The listing builds one solid part. Answer for the finished solid, in the listing's coordinates (mm). A direction names the side the tool comes from. Give positions to 0.01 mm unless a question says otherwise; leave off trailing zeros. Write each loop counter-clockwise with the first axis right and the second up, starting at its lowest first coordinate (ties: lowest second). Pieces come first, ordered by that corner, then holes.
```python
from build123d import *

# Parameters (mm, degrees)
F1_DEPTH = 6
F2_R     = 6.25
F3_DEPTH = 3.5
F4_W     = 15.8
F4_H     = 32
F5_DEPTH = 4.5
F7_DEPTH = 32
F9_DEPTH = 15.8
F10_R    = 0.2


with BuildPart() as f1:
    # F0 (on Top) → F1 (new body)
    with BuildSketch(Plane.XY):
        with BuildLine():
            ThreePointArc((-29.927051, 63.999335), (-26.535898, 58), (-33.427051, 57.937157))
            Line((-33.427051, 57.937157), (-37.47822, 60.2761))
            ThreePointArc((-37.47822, 60.2761), (-38.509832, 60.257063), (-38.975497, 59.336334))
            ThreePointArc((-38.975497, 59.336334), (-38.676985, 57.610456), (-38.049845, 55.975078))
            Line((-38.049845, 55.975078), (-8.049845, -4.024922))
            ThreePointArc((-8.049845, -4.024922), (-6.775035, -5.924433), (-5.0625, -7.441176))
            ThreePointArc((-5.0625, -7.441176), (-4.032293, -7.498262), (-3.5, -6.614378))
            Line((-3.5, -6.614378), (-3.5, -1.936492))
            ThreePointArc((-3.5, -1.936492), (0, 4), (3.5, -1.936492))
            Line((3.5, -1.936492), (3.5, -6.614378))
            ThreePointArc((3.5, -6.614378), (4.032293, -7.498262), (5.0625, -7.441176))
            ThreePointArc((5.0625, -7.441176), (6.775035, -5.924433), (8.049845, -4.024922))
            Line((8.049845, -4.024922), (38.049845, 55.975078))
            ThreePointArc((38.049845, 55.975078), (38.676985, 57.610456), (38.975497, 59.336334))
            ThreePointArc((38.975497, 59.336334), (38.509832, 60.257063), (37.47822, 60.2761))
            Line((37.47822, 60.2761), (33.427051, 57.937157))
            ThreePointArc((33.427051, 57.937157), (26.535898, 58), (29.927051, 63.999335))
            Line((29.927051, 63.999335), (33.97822, 66.338278))
            ThreePointArc((33.97822, 66.338278), (34.477539, 67.241199), (33.912997, 68.104841))
            ThreePointArc((33.912997, 68.104841), (32.007041, 68.773357), (30, 69))
            Line((30, 69), (-30, 69))
            ThreePointArc((-30, 69), (-32.007041, 68.773357), (-33.912997, 68.104841))
            ThreePointArc((-33.912997, 68.104841), (-34.477539, 67.241199), (-33.97822, 66.338278))
            Line((-33.97822, 66.338278), (-29.927051, 63.999335))
        make_face()
    extrude(amount=F1_DEPTH)

    # F2 (on face) → F3 (cut)
    with BuildSketch(Plane.XY.offset(6)):
        with Locations((-30, 60)):
            Circle(F2_R)
        Circle(F2_R)
        with Locations((30, 60)):
            Circle(F2_R)
    extrude(amount=-F3_DEPTH, mode=Mode.SUBTRACT)

    # F4 (on face) → F5 (join)
    with BuildSketch(Plane.XY.offset(6)):
        with Locations((0, 31)):
            Rectangle(F4_W, F4_H)
    extrude(amount=F5_DEPTH)

    # F6 (on face) → F7 (join)
    with BuildSketch(Plane.XZ.offset(-15)):
        Polygon((9, 10.5), (7.9, 10.5), (7.9, 8.594744), align=None)
        Polygon((-7.9, 8.594744), (-7.9, 10.5), (-9, 10.5), align=None)
    extrude(amount=-F7_DEPTH)

    # F8 (on face) → F9 (join)
    with BuildSketch(Plane(origin=(-7.9, 0, 0), x_dir=(0, -1, 0), z_dir=(-1, 0, 0))):
        Polygon((-6.5, 6), (-15, 8.594744), (-15, 6), align=None)
        Polygon((-47, 6), (-47, 8.594744), (-53.5, 6), align=None)
    extrude(amount=-F9_DEPTH)

    # F10
    f10_edges = [f1.edges().sort_by_distance(p)[0] for p in [
        (-9, 31, 10.5),
        (9, 31, 10.5),
        (0, 15, 10.5),
        (0, 47, 10.5),
    ]]
    fillet(f10_edges, radius=F10_R)


solid = f1.part
```
Item 1: A cutting plane is placed at B-B, the plane z = 1.5. Give the vertices of the cut face in (x, y).
Conclusion:
outline: (-38.98, 59.34) arc R9 ccw to (-38.05, 55.98) - (-8.05, -4.02) arc R9 ccw to (-5.06, -7.44) arc R1 ccw to (-3.5, -6.61) - (-3.5, -1.94) arc R4 cw (long way) to (3.5, -1.94) - (3.5, -6.61) arc R1 ccw to (5.06, -7.44) arc R9 ccw to (8.05, -4.02) - (38.05, 55.98) arc R9 ccw to (38.98, 59.34) arc R1 ccw to (37.48, 60.28) - (33.43, 57.94) arc R4 cw (long way) to (29.93, 64) - (33.98, 66.34) arc R1 ccw to (33.91, 68.1) arc R9 ccw to (30, 69) - (-30, 69) arc R9 ccw to (-33.91, 68.1) arc R1 ccw to (-33.98, 66.34) - (-29.93, 64) arc R4 cw (long way) to (-33.43, 57.94) - (-37.48, 60.28) arc R1 ccw to start
Item 2: A cutting plane is placed at C-C, the plane x = 0. Give the vertices of the cut face in (y, z).
Conclusion:
outline: (4, 0) - (69, 0) - (69, 6) - (53.5, 6) - (47, 8.59) - (47, 10.3) arc R0.2 ccw to (46.8, 10.5) - (15.2, 10.5) arc R0.2 ccw to (15, 10.3) - (15, 8.59) - (6.5, 6) - (6.25, 6) - (6.25, 2.5) - (4, 2.5) - close
Item 3: A cutting plane is placed at D-D, the plane x = -29. Give the vertices of the cut face in (y, z).
Conclusion:
outline: (37.88, 0) - (56.13, 0) - (56.13, 2.5) - (53.83, 2.5) - (53.83, 6) - (37.88, 6) - close; (63.87, 0) - (69, 0) - (69, 6) - (66.17, 6) - (66.17, 2.5) - (63.87, 2.5) - close
Item 4: Consider probe 1 along X at (y, z) = (60, 5.2); probe 2 along X at (y, z) = (60, 0.95); probe 3 along Z at (x, y) = (17, 60). Determine where each line is inside the solid, lowest interval first.
Conclusion:
probe 1: x = -38.79 to -37, -23.75 to 23.75, 37 to 38.79
probe 2: x = -38.79 to -37, -26 to 26, 37 to 38.79
probe 3: z = 0 to 6
Item 5: Determine the mould class of faces 5 (the face through (-26.48, 58.1, 1.23)), 6 (the face through (-0.111, 50.204, 7.316)), 7 (the face through (34.478, 67.226, 2.958)) for opening direction X: pulls with the +X half, pulls with the -X half, needs draft (parallel to the pull), parting line crosses it, or undercut.
Conclusion:
face 5: undercut
face 6: needs draft
face 7: pulls with the +X half
Item 6: A cutting plane is placed at A-A, the plane y = 2. Give the vertices of the cut face in (x, z).
Conclusion:
outline: (-11.06, 0) - (-3.46, 0) - (-3.46, 2.5) - (-5.92, 2.5) - (-5.92, 6) - (-11.06, 6) - close; (3.46, 0) - (11.06, 0) - (11.06, 6) - (5.92, 6) - (5.92, 2.5) - (3.46, 2.5) - close
Item 7: Each of these flat-tipped pins is pushed along its axis until it touches: P1, Ø1.4, axis at y = -4, z = 4, coming from the -X side; P2, Ø2, axis at x = 0.5, y = 49, coming from the -Z side; P3, Ø4, axis at y = 4.5, z = 4.5, coming from the +X side; P4, Ø14.5, axis at x = 30, y = 60, coming from the +Z side. Where does it stop, or does it pass through?
Conclusion:
P1: stops at x = -8.41
P2: stops at z = 0
P3: stops at x = 13.31
P4: stops at z = 6
Item 8: Which of the six approach directions +Z, -Z, +X, -X, +Y, -Y give full straight-line access (tool end or side, diameter ignored) to faces 1 (the face through (-25.9, 58.7, 2.5)), 2 (the face through (-35.874, 59.35, 2.291)), 3 (the face through (-7.9, 30, 7)), 4 (the face through (7.9, 30, 7))?
Conclusion:
face 1: +Z
face 2: +Z, -Z
face 3: -X, +Y, -Y
face 4: +X, +Y, -Y
